```python
from build123d import *

# Parameters (mm, degrees)
BOSS_EXTRUDE1_DEPTH = 3.175
CUT_EXTRUDE1_DEPTH  = 4.175


with BuildPart() as part:
    # Sketch1 → Boss-Extrude1 (new body)
    with BuildSketch(Plane.XY):
        Polygon((-950.530495659, 69.619322302), (-951.061849964, 63.291592645), (-11.536706102, -24.902638492), (-8.372841274, -25.168315645), (0, -25.545856054), (152.4, -25.545856054), (152.4, -7.765856054), (139.7, -7.765856054), (139.7, -12.845856054), (136.525, -12.845856054), (136.525, -7.765856054), (95.25, -7.765856054), (95.25, -12.845856054), (92.075, -12.845856054), (92.075, -7.765856054), (79.375, -7.765856054), (79.375, -12.845856054), (76.2, -12.845856054), (76.2, -7.765856054), (69.85, -7.765856054), (25.4, -0.145856054), (19.05, -0.145856054), (19.05, -5.225856054), (15.875, -5.225856054), (15.875, -0.145856054), (3.175, -0.145856054), (3.175, -6.495856054), (0, -6.495856054), (0, -0.145856054), (-2.81225704, -0.145856054), (-6.247424053, 0.14260298), (-6.778778359, -6.185126677), (-9.942643187, -5.919449524), (-9.411288881, 0.408280132), (-946.54805097, 79.101852726), (-947.366630831, 69.353645149), align=None)
    extrude(amount=BOSS_EXTRUDE1_DEPTH)

    # Sketch2 → Cut-Extrude1 (cut, through all)
    with BuildSketch(Plane.XY.offset(3.175)):
        Polygon((-79.415081651, -0.013332249), (-78.889760507, 6.242550403), (-82.053625335, 6.508227555), (-82.578671745, 0.255616625), align=None)
        Polygon((-158.378290396, 6.699631648), (-157.859826617, 12.873852131), (-161.023691445, 13.139529284), (-161.54188049, 6.968580522), align=None)
        Polygon((-237.341499142, 13.412595546), (-236.829892727, 19.50515386), (-239.993757555, 19.770831012), (-240.505089236, 13.68154442), align=None)
        Polygon((-316.304707888, 20.125559443), (-315.799958836, 26.136455588), (-318.963823664, 26.402132741), (-319.468297982, 20.394508317), align=None)
        Polygon((-395.267916634, 26.83852334), (-394.770024946, 32.767757316), (-397.933889774, 33.033434469), (-398.431506728, 27.107472214), align=None)
        Polygon((-474.23112538, 33.551487238), (-473.740091056, 39.399059045), (-476.903955884, 39.664736197), (-477.394715474, 33.820436112), align=None)
        Polygon((-553.194334126, 40.264451135), (-552.710157166, 46.030360773), (-555.874021994, 46.296037926), (-556.35792422, 40.533400009), align=None)
        Polygon((-632.157542872, 46.977415032), (-631.680223276, 52.661662502), (-634.844088104, 52.927339654), (-635.321132966, 47.246363906), align=None)
        Polygon((-711.120751618, 53.69037893), (-710.650289385, 59.29296423), (-713.814154213, 59.558641383), (-714.284341712, 53.959327804), align=None)
        Polygon((-790.083960364, 60.403342827), (-789.620355495, 65.924265958), (-792.784220323, 66.189943111), (-793.247550458, 60.672291701), align=None)
        Polygon((-869.047169109, 67.116306724), (-868.590421605, 72.555567687), (-871.754286433, 72.821244839), (-872.210759203, 67.385255598), align=None)
    extrude(amount=-CUT_EXTRUDE1_DEPTH, mode=Mode.SUBTRACT)


solid = part.part
```
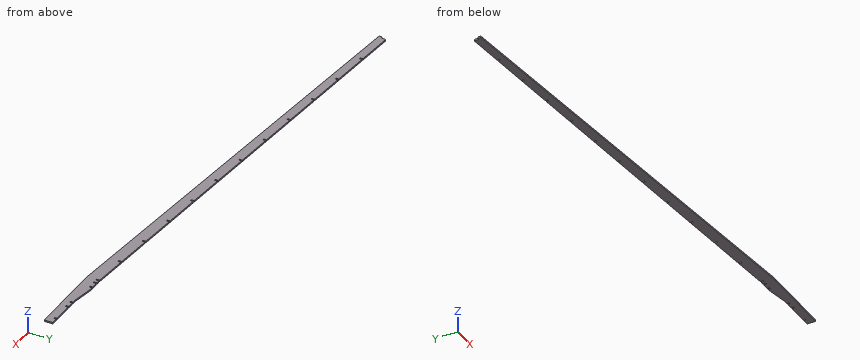
The listing builds one solid part. Answer for the finished solid, in the listing's coordinates (mm). Coordinates: 2 decimals unless noted, no trailing zeros. Write each loop counter-clockwise with the first axis right and the second up, starting at its lowest first coordinate (ties: lowest second). Pieces come first, ordered by that corner, then holes. Notation, with made-up numbers: (87, -10.75) - (107, -10.75) arc R18 cw to (107, 24.25) - close; hole circle Ø5 at (-16, -27). An arc over 180 degrees is marked (long way). Return JSON: item names as keys, results as strings. Group by question number.
Q1. The part is cut by section B-B on x = -139. Write down the section's boundary in (y, z) (3 decimals).
Q2. Flat-ended cylindrical pins translate along their axes: pin 1 Ø1 at (x, z) = (1, 2.5) entering from +Y; pin 2 Ø1.6 at (x, z) = (83, 2) entering from +Y; pin 3 Ø1 at (x, z) = (77, 2) entering from +Y. Find the tip coordinate at first contact, or state that the pin passes through.
Q3. The part is cut by section A-A on x = -443. Write down the section's boundary in (y, z) (3 decimals), and give its area (3 significant figures).
Q4. Find the intervals of material crossed by line 1 along Y through (x, z) = (-202, 0.85); line 2 along Y through (x, z) = (-446, 2.5), in increasing order. Write a range as [from, to].
Evaluation:
{
 "1": {"outline": "(-12.938, 0) - (11.29, 0) - (11.29, 3.175) - (-12.938, 3.175) - close"},
 "2": {"pin 1": "stops at y = -6.5", "pin 2": "stops at y = -7.77", "pin 3": "stops at y = -12.85"},
 "3": {"outline": "(15.599, 0) - (36.818, 0) - (36.818, 3.175) - (15.599, 3.175) - close", "area": "67.4 mm2"},
 "4": {"line 1": "y = [-7.02, 16.58]", "line 2": "y = [15.88, 37.07]"}
}
